from build123d import *

# Parameters (mm, degrees)
SKETCH1_W           = 152.4
SKETCH1_H           = 127
BOSS_EXTRUDE1_DEPTH = 76.2
CUT_EXTRUDE1_DEPTH  = 182.836327504
SKETCH3_W           = 123.769027692
SKETCH3_H           = 102.663904472
CUT_EXTRUDE2_DEPTH  = 182.836327504
SKETCH4_R           = 46.960856135
CUT_EXTRUDE3_DEPTH  = 167.558938517


with BuildPart() as part:
    # Sketch1 → Boss-Extrude1 (new, symmetric)
    with BuildSketch(Plane.XY):
        Rectangle(SKETCH1_W, SKETCH1_H)
    extrude(amount=BOSS_EXTRUDE1_DEPTH, both=True)

    # Sketch2 → Cut-Extrude1 (cut, through all)
    with BuildSketch(Plane.XY.offset(76.2)):
        Polygon((0, 50.550598249), (-43.77810226, -25.275299124), (43.77810226, -25.275299124), align=None)
    extrude(amount=-CUT_EXTRUDE1_DEPTH, mode=Mode.SUBTRACT)

    # Sketch3 → Cut-Extrude2 (cut, through all)
    with BuildSketch(Plane(origin=(76.2, 0, 0), x_dir=(0, 0, -1), z_dir=(1, 0, 0))):
        Rectangle(SKETCH3_W, SKETCH3_H)
    extrude(amount=-CUT_EXTRUDE2_DEPTH, mode=Mode.SUBTRACT)

    # Sketch4 → Cut-Extrude3 (cut, through all)
    with BuildSketch(Plane(origin=(0, 63.5, 0), x_dir=(1, 0, 0), z_dir=(0, 1, 0))):
        with Locations(Location((0, 0, 0), (0, 0, 270))):
            Circle(SKETCH4_R)
    extrude(amount=-CUT_EXTRUDE3_DEPTH, mode=Mode.SUBTRACT)


solid = part.part
Build history of the part. All positions in model axes, mm. A direction names the side the tool comes from. Give positions to 0.01 mm unless a question says otherwise; leave off trailing zeros. Loops run counter-clockwise (first coordinate to the right, second up) from the corner with the lowest first, then second, coordinate; pieces in that order, holes last. Notation, with made-up numbers: (41, 56) -> (52, 56) arc R11 cw to (52, 67) -> close; hole circle Ø11 at (21.25, 76.25). An arc over 180 degrees is marked (long way). Answer in a Markdown table with one row per item.
Item 1: Slice it at C-C on x = 58.5. Write the cut outline in (y, z).
Findings below:
| item | result |
|---|---|
| outline | (-63.5, -76.2) -> (63.5, -76.2) -> (63.5, 76.2) -> (-63.5, 76.2) -> close; hole (-51.33, -61.88) -> (51.33, -61.88) -> (51.33, 61.88) -> (-51.33, 61.88) -> close |
Item 2: Tool access for faces 1 (the flat face through (-1, -25.275, 69)), 2 (the flat face through (-1, -27, 76.2)), 3 (the flat face through (18, 22, 61.885)): list every direction of +Z, -Z, +X, -X, +Y, -Y with a clear straight run to the whole face (end or side of a thin tool).
Findings below:
| item | result |
|---|---|
| face 1 | +Z, -Z |
| face 2 | +Z, +X, -X, +Y, -Y |
| face 3 | +X, -X |
Item 3: Slice it at A-A on y = -35. Write the cut outline in (x, z).
Findings below:
| item | result |
|---|---|
| outline | (-76.2, -76.2) -> (76.2, -76.2) -> (76.2, -61.88) -> (-76.2, -61.88) -> close; (-76.2, 61.88) -> (76.2, 61.88) -> (76.2, 76.2) -> (-76.2, 76.2) -> close |
Item 4: Mould opens along X. For faces 4 (the flat face through (76.2, -57, 1)), 5 (the cylindrical face through (-45.844, 57.501, -10.18)), 6 (the flat face through (-1, -27, -76.2)), 7 (the flat face through (22.2, 12.1, -68.9)) say: pulls with the +X half, pulls with the -X half, needs draft (parallel to the pull), parting line crosses it, or undercut.
Findings below:
| item | result |
|---|---|
| face 4 | pulls with the +X half |
| face 5 | undercut |
| face 6 | needs draft |
| face 7 | undercut |
Item 5: Slice it at B-B on z = 51. Write the cut outline in (x, y), plus the area to 3 significant figures.
Findings below:
| item | result |
|---|---|
| outline | (-76.2, -63.5) -> (76.2, -63.5) -> (76.2, -51.33) -> (-76.2, -51.33) -> close; (-76.2, 51.33) -> (76.2, 51.33) -> (76.2, 63.5) -> (-76.2, 63.5) -> close |
| area | 3,710 mm² |
Item 6: Slice it at D-D on z = 0. Write the cut outline in (x, y), plus the area to 3 significant figures.
Findings below:
| item | result |
|---|---|
| outline | (-76.2, -63.5) -> (-46.96, -63.5) -> (-46.96, -51.33) -> (-76.2, -51.33) -> close; (-76.2, 51.33) -> (-46.96, 51.33) -> (-46.96, 63.5) -> (-76.2, 63.5) -> close; (46.96, -63.5) -> (76.2, -63.5) -> (76.2, -51.33) -> (46.96, -51.33) -> close; (46.96, 51.33) -> (76.2, 51.33) -> (76.2, 63.5) -> (46.96, 63.5) -> close |
| area | 1,420 mm² |
Item 7: Probe line 1 along Y through (x, z) = (26, -40); line 2 along Z through (x, y) = (60, 17); line 3 along X through (y, z) = (-57.25, 0). List the from-to ranges inside material, lowest first. Write a range as [from, to].
Findings below:
| item | result |
|---|---|
| line 1 | y = [-63.5, -51.33], [51.33, 63.5] |
| line 2 | z = [-76.2, -61.88], [61.88, 76.2] |
| line 3 | x = [-76.2, -46.96], [46.96, 76.2] |
Item 8: Flat gauge pin, fed straight in: P1, Ø8, axis at x = -12, y = 15, coming from the +Z side. Where does the tip first touch, or does it go through?
Findings below:
| item | result |
|---|---|
| P1 | passes through |
